Autodesk Fusion 360 part; units mm, degrees
sketch "Sketch1" plane through (0, 0, 0) normal (0, 0, 1) x (1, 0, 0)
  line L0 (85.6912, 5) -> (85.6912, 58)
  line L1 (55.6912, 58) -> (55.6912, 5)
  line L2 (80.6912, 0) -> (80.6912, 8)
  line L3 (80.6912, 8) -> (60.6912, 8)
  line L4 (60.6912, 8) -> (60.6912, 0)
  line L5 (78.6912, 65) -> (62.6912, 65)
  line L6 (50.6912, 0) -> (60.6912, 0)
  circle A0 centre (70.6912, 47.793) radius 5
  line L7 (70.6912, 65) -> (70.6912, 26.651) construction
  line L8 (50.6912, 0) -> (50.6912, 5)
  line L9 (55.6912, 13.8) -> (85.6912, 13.8)
  line L10 (90.6912, 5) -> (90.6912, 0)
  line L11 (90.6912, 0) -> (80.6912, 0)
  line L12 (50.6912, 5) -> (55.6912, 5)
  line L13 (85.6912, 5) -> (90.6912, 5)
  arc A1 (62.6912, 65) -> (55.6912, 58) centre (62.6912, 58) ccw
  arc A2 (85.6912, 58) -> (78.6912, 65) centre (78.6912, 58) ccw
  dimension "d1" = 20
  dimension "d2" = 8
  dimension "d9" = 10
  dimension "d12" = 5.8
  dimension "d13" = 10
  dimension "d14" = 10
  dimension "d15" = 5
  dimension "d16" = 5
  dimension "d17" = 5
  dimension "d18" = 5
  dimension "d19" = 47.793
  dimension "d20" = 65
  dimension "d21" = 7
extrude "Extrude1" add sketch "Sketch1" along normal blind 5 contours L0 L1 L5 L9 A1 A2
extrude "Extrude2" add sketch "Sketch1" along normal blind 30 contours L0 L1 L2 L3 L4 L6 L8 L9 L10 L11 L12 L13
sketch "Sketch2" plane through (0, 13.8, 0) normal (0, 1, 0) x (-1, 0, 0)
  line L0 (-85.6912, 5) -> (-55.6912, 5)
  line L1 (-55.6912, 5) -> (-55.6912, 30)
  line L2 (-55.6912, 30) -> (-85.6912, 30)
  line L3 (-85.6912, 30) -> (-85.6912, 5)
  line L4 (-63.185, 12.5052) -> (-78.185, 12.5052) construction
  line L5 (-78.185, 12.5052) -> (-78.185, 22.5052) construction
  line L6 (-78.185, 22.5052) -> (-63.185, 22.5052) construction
  line L7 (-63.185, 22.5052) -> (-63.185, 12.5052) construction
  line L8 (-70.685, 17.4948) -> (-70.685, 17.5052)
  circle A0 centre (-63.185, 12.5052) radius 1.5
  circle A1 centre (-78.185, 12.5052) radius 1.5
  circle A2 centre (-78.185, 22.5052) radius 1.5
  circle A3 centre (-63.185, 22.5052) radius 1.5
  dimension "d26" = 15
  dimension "d27" = 10
  dimension "d28" = 3
extrude "Extrude3" cut sketch "Sketch2" along normal through all contours A0 | A1 | A2 | A3
Could you check a few things on this model? Use its own coordinates, in mm. A direction names the side the tool comes from. Round coordinates to 2 decimals unless told otherwise and drop trailing zeros. Write each loop counter-clockwise with the first axis right and the second up, starting at its lowest first coordinate (ties: lowest second). Pieces come first, ordered by that corner, then holes. Notation, with made-up numbers: (52.5, 71) -> (86.5, 71) arc R29 ccw to (86.5, 106) -> close; hole circle Ø7 at (-9.5, 79). An arc over 180 degrees is marked (long way). Use a Markdown table: item, result.
1. If we section it at A-A (y = 6): List the corners of the cut face in (x, z) for me.
Answer key:
| item | result |
|---|---|
| outline | (55.69, 0) -> (60.69, 0) -> (60.69, 30) -> (55.69, 30) -> close; (80.69, 0) -> (85.69, 0) -> (85.69, 30) -> (80.69, 30) -> close |
2. Please list where these lines run through material, in increasing order: probe 1 along X at (y, z) = (6.5, 5.75); probe 2 along Z at (x, y) = (60, 26); probe 3 along X at (y, z) = (16, 3).
Answer key:
| item | result |
|---|---|
| probe 1 | x = 55.69 to 60.69, 80.69 to 85.69 |
| probe 2 | z = 0 to 5 |
| probe 3 | x = 55.69 to 85.69 |
3. If we section it at D-D (x = 65): List the corners of the cut face in (y, z) for me, then the cut area to 3 significant figures.
Answer key:
| item | result |
|---|---|
| outline | (8, 0) -> (65, 0) -> (65, 5) -> (13.8, 5) -> (13.8, 30) -> (8, 30) -> close |
| area | 430 mm^2 |
4. If we section it at C-C (z = 13.75): List the corners of the cut face in (x, y) for me, then the cut area to 3 significant figures.
Answer key:
| item | result |
|---|---|
| outline | (50.69, 0) -> (60.69, 0) -> (60.69, 8) -> (80.69, 8) -> (80.69, 0) -> (90.69, 0) -> (90.69, 5) -> (85.69, 5) -> (85.69, 13.8) -> (55.69, 13.8) -> (55.69, 5) -> (50.69, 5) -> close |
| area | 304 mm^2 |
5. We'd pull the mould along X, two halves only. Please class faces 5 (the face through (83.59, 63, 2.46)), 6 (the face through (70, 40, 5)), 7 (the face through (60.691, 4, 15)): +X half, -X half, draft (parallel to the pull), parting line (faces both ways), or undercut.
Answer key:
| item | result |
|---|---|
| face 5 | +X half |
| face 6 | draft |
| face 7 | undercut |
6. Which directions (+Z, -Z, +X, -X, +Y, -Y) give clear straight access to the entire face, cutting with the end or side of a thin tool? Please do faces 1 (the face through (71, 8, 15)), 2 (the face through (70, 13.8, 17)), 3 (the face through (55.691, 24, 3)), 4 (the face through (85.691, 19.4, 4.8)).
Answer key:
| item | result |
|---|---|
| face 1 | +Z, -Z, -Y |
| face 2 | +Z, +X, -X, +Y |
| face 3 | +Z, -Z, -X, +Y |
| face 4 | +Z, -Z, +X, +Y |
7. If we section it at B-B (x = 70.5): List the corners of the cut face in (y, z) for me.
Answer key:
| item | result |
|---|---|
| outline | (8, 0) -> (42.8, 0) -> (42.8, 5) -> (13.8, 5) -> (13.8, 30) -> (8, 30) -> close; (52.79, 0) -> (65, 0) -> (65, 5) -> (52.79, 5) -> close |
8. For pin 1 Ø15 at (y, z) = (22.5, 16.5) entering from -X; pin 2 Ø8 at (x, z) = (79.5, 13.5) entering from +Y; pin 3 Ø10 at (x, y) = (57, 17.5) entering from -Z; pin 4 Ø2 at (y, z) = (8.5, 10.5) entering from -X, each with a flat end and sliding along its axis, tell me the tip position at first contact or that it passes through.
Answer key:
| item | result |
|---|---|
| pin 1 | passes through |
| pin 2 | stops at y = 13.8 |
| pin 3 | stops at z = 0 |
| pin 4 | stops at x = 55.69 |
